The figure shows three views and two pictorial views of one solid part (mm, origin at its lowest corner). Answer the questions. Coordinates: 2 decimals unless noted, no trailing zeros. Write each loop counter-clockwise with the first axis right and the second up, starting at its lowest first coordinate (ties: lowest second). Pieces come first, ordered by that corner, then holes.
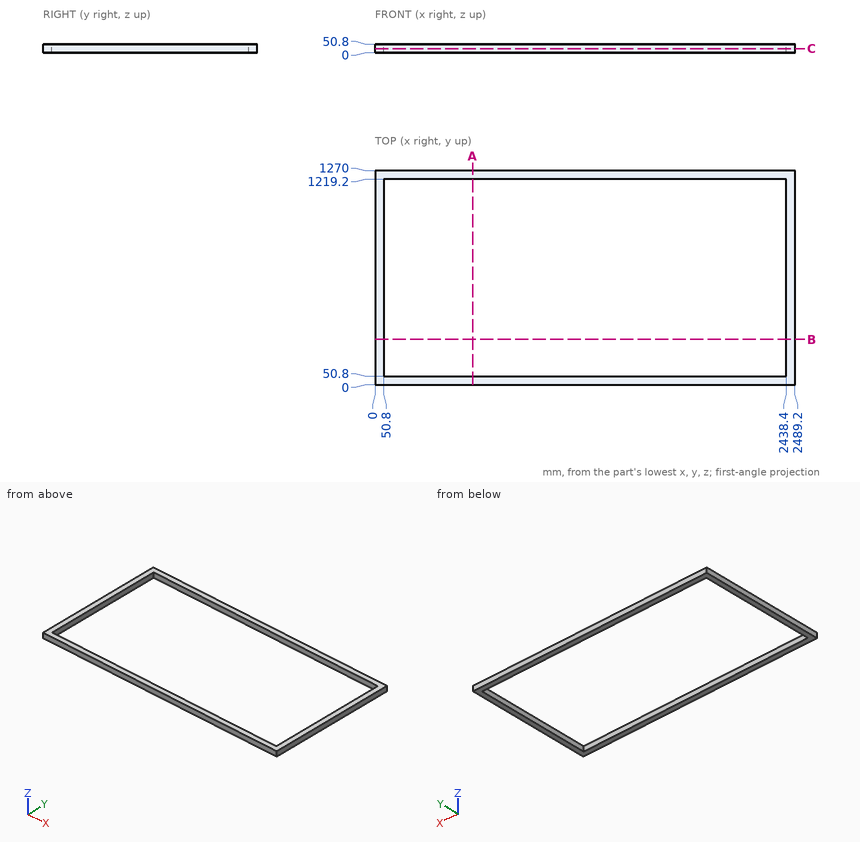
Item 1: The part is cut by section A-A (x = 578). Give the vertices of the cut face in (y, z), and give its area (3 significant figures).
Item 2: Find the intervals of material crossed by probe 1 along X at (y, z) = (788.5, 37); probe 2 along Y at (x, z) = (936, 27), in increasing order.
Item 3: The part is cut by section C-C (z = 23.5). Give the vertices of the cut face in (x, y).
Item 4: The part is cut by section B-B (y = 269). Give the vertices of the cut face in (x, z).
Answer:
1. outline: (0, 0) - (50.8, 0) - (50.8, 50.8) - (0, 50.8) - close; (1219.2, 0) - (1270, 0) - (1270, 50.8) - (1219.2, 50.8) - close
1. area: 5,160 mm2
2. probe 1: x = 0 to 50.8, 2438.4 to 2489.2
2. probe 2: y = 0 to 50.8, 1219.2 to 1270
3. outline: (0, 0) - (2489.2, 0) - (2489.2, 1270) - (0, 1270) - close; hole (50.8, 50.8) - (2438.4, 50.8) - (2438.4, 1219.2) - (50.8, 1219.2) - close
4. outline: (0, 0) - (50.8, 0) - (50.8, 50.8) - (0, 50.8) - close; (2438.4, 0) - (2489.2, 0) - (2489.2, 50.8) - (2438.4, 50.8) - close
